Geometry check sheet. Reference: the model listing, model coordinates, mm. Give positions to 0.01 mm unless a question says otherwise; leave off trailing zeros. Write each loop counter-clockwise with the first axis right and the second up, starting at its lowest first coordinate (ties: lowest second). Pieces come first, ordered by that corner, then holes. Notation, with made-up numbers: (45, 46.5) -> (49, 46.5) arc R23 cw to (49, 84.5) -> close; hole circle Ø6 at (68, -35.5). An arc over 180 degrees is marked (long way). Write item = value, one per line. Start each with the question number.
1. Depth check by flat-ended pin: P1, Ø1.5, axis at x = -33, z = 1.5, coming from the +Y side; P2, Ø1.5, axis at x = -59, z = 1, coming from the -Y side. Enter the tip coordinate at first touch or a pass-through.
2. Cross-section at C-C, the plane z = 2.1. State how many separate pieces and enclosed holes the cut face has, plus the area to 3 significant figures.
3. Cross-section at B-B, the plane x = 27.5. Record the cut outline in (y, z).
4. Thickness scan on line 1 along X through (y, z) = (45.5, 0.8); line 2 along Y through (x, z) = (23.5, 2.65). Record the ranges inside material, lowest first.
5. Cross-section at A-A, the plane y = -53. Record the cut outline in (x, z), plus the area to 3 significant figures.
Autodesk Inventor part; units mm, degrees
ref_plane "YZ Plane" through (0, 0, 0) normal (1, 0, 0) x (0, 1, 0)
ref_plane "XZ Plane" through (0, 0, 0) normal (0, 1, 0) x (-1, 0, 0)
ref_plane "XY Plane" through (0, 0, 0) normal (0, 0, 1) x (1, 0, 0)
sketch "Sketch1" plane through (0, 0, 0) normal (0, 0, 1) x (1, 0, 0)
  line L0 (-65, -90.5) -> (65, -90.5)
  line L1 (65, -90.5) -> (65, 90.5)
  line L2 (65, 90.5) -> (-65, 90.5)
  line L3 (-65, 90.5) -> (-65, -90.5)
  line L4 (-65, -90.5) -> (65, 90.5) construction
  line L5 (65, -90.5) -> (-65, 90.5) construction
  line L6 (-60, 77.5) -> (-57, 77.5)
  line L7 (-57, 77.5) -> (-57, 62.5)
  line L8 (-57, 62.5) -> (-60, 62.5)
  line L9 (-60, 62.5) -> (-60, 77.5)
  line L10 (-60, 77.5) -> (-57, 62.5) construction
  line L11 (-57, 77.5) -> (-60, 62.5) construction
  line L12 (-60, 57.5) -> (-57, 57.5)
  line L13 (-57, 57.5) -> (-57, 42.5)
  line L14 (-57, 42.5) -> (-60, 42.5)
  line L15 (-60, 42.5) -> (-60, 57.5)
  line L16 (-60, 57.5) -> (-57, 42.5) construction
  line L17 (-57, 57.5) -> (-60, 42.5) construction
  line L18 (-60, 37.5) -> (-57, 37.5)
  line L19 (-57, 37.5) -> (-57, 22.5)
  line L20 (-57, 22.5) -> (-60, 22.5)
  line L21 (-60, 22.5) -> (-60, 37.5)
  line L22 (-60, 37.5) -> (-57, 22.5) construction
  line L23 (-57, 37.5) -> (-60, 22.5) construction
  line L24 (-60, 17.5) -> (-57, 17.5)
  line L25 (-57, 17.5) -> (-57, 2.5)
  line L26 (-57, 2.5) -> (-60, 2.5)
  line L27 (-60, 2.5) -> (-60, 17.5)
  line L28 (-60, 17.5) -> (-57, 2.5) construction
  line L29 (-57, 17.5) -> (-60, 2.5) construction
  line L30 (-60, -2.5) -> (-57, -2.5)
  line L31 (-57, -2.5) -> (-57, -17.5)
  line L32 (-57, -17.5) -> (-60, -17.5)
  line L33 (-60, -17.5) -> (-60, -2.5)
  line L34 (-60, -2.5) -> (-57, -17.5) construction
  line L35 (-57, -2.5) -> (-60, -17.5) construction
  line L36 (-60, -22.5) -> (-57, -22.5)
  line L37 (-57, -22.5) -> (-57, -37.5)
  line L38 (-57, -37.5) -> (-60, -37.5)
  line L39 (-60, -37.5) -> (-60, -22.5)
  line L40 (-60, -22.5) -> (-57, -37.5) construction
  line L41 (-57, -22.5) -> (-60, -37.5) construction
  line L42 (-60, -42.5) -> (-57, -42.5)
  line L43 (-57, -42.5) -> (-57, -57.5)
  line L44 (-57, -57.5) -> (-60, -57.5)
  line L45 (-60, -57.5) -> (-60, -42.5)
  line L46 (-60, -42.5) -> (-57, -57.5) construction
  line L47 (-57, -42.5) -> (-60, -57.5) construction
  line L48 (-60, -62.5) -> (-57, -62.5)
  line L49 (-57, -62.5) -> (-57, -77.5)
  line L50 (-57, -77.5) -> (-60, -77.5)
  line L51 (-60, -77.5) -> (-60, -62.5)
  line L52 (-60, -62.5) -> (-57, -77.5) construction
  line L53 (-57, -62.5) -> (-60, -77.5) construction
  line L54 (57, 77.5) -> (60, 77.5)
  line L55 (60, 77.5) -> (60, 62.5)
  line L56 (60, 62.5) -> (57, 62.5)
  line L57 (57, 62.5) -> (57, 77.5)
  line L58 (57, 77.5) -> (60, 62.5) construction
  line L59 (60, 77.5) -> (57, 62.5) construction
  line L60 (57, 57.5) -> (60, 57.5)
  line L61 (60, 57.5) -> (60, 42.5)
  line L62 (60, 42.5) -> (57, 42.5)
  line L63 (57, 42.5) -> (57, 57.5)
  line L64 (57, 57.5) -> (60, 42.5) construction
  line L65 (60, 57.5) -> (57, 42.5) construction
  line L66 (57, 37.5) -> (60, 37.5)
  line L67 (60, 37.5) -> (60, 22.5)
  line L68 (60, 22.5) -> (57, 22.5)
  line L69 (57, 22.5) -> (57, 37.5)
  line L70 (57, 37.5) -> (60, 22.5) construction
  line L71 (60, 37.5) -> (57, 22.5) construction
  line L72 (57, 17.5) -> (60, 17.5)
  line L73 (60, 17.5) -> (60, 2.5)
  line L74 (60, 2.5) -> (57, 2.5)
  line L75 (57, 2.5) -> (57, 17.5)
  line L76 (57, 17.5) -> (60, 2.5) construction
  line L77 (60, 17.5) -> (57, 2.5) construction
  line L78 (57, -2.5) -> (60, -2.5)
  line L79 (60, -2.5) -> (60, -17.5)
  line L80 (60, -17.5) -> (57, -17.5)
  line L81 (57, -17.5) -> (57, -2.5)
  line L82 (57, -2.5) -> (60, -17.5) construction
  line L83 (60, -2.5) -> (57, -17.5) construction
  line L84 (57, -22.5) -> (60, -22.5)
  line L85 (60, -22.5) -> (60, -37.5)
  line L86 (60, -37.5) -> (57, -37.5)
  line L87 (57, -37.5) -> (57, -22.5)
  line L88 (57, -22.5) -> (60, -37.5) construction
  line L89 (60, -22.5) -> (57, -37.5) construction
  line L90 (57, -42.5) -> (60, -42.5)
  line L91 (60, -42.5) -> (60, -57.5)
  line L92 (60, -57.5) -> (57, -57.5)
  line L93 (57, -57.5) -> (57, -42.5)
  line L94 (57, -42.5) -> (60, -57.5) construction
  line L95 (60, -42.5) -> (57, -57.5) construction
  line L96 (57, -62.5) -> (60, -62.5)
  line L97 (60, -62.5) -> (60, -77.5)
  line L98 (60, -77.5) -> (57, -77.5)
  line L99 (57, -77.5) -> (57, -62.5)
  line L100 (57, -62.5) -> (60, -77.5) construction
  line L101 (60, -62.5) -> (57, -77.5) construction
  point P0 (0, 0)
  point P1 (-58.5, 70)
  point P2 (-58.5, 50)
  point P3 (-58.5, 30)
  point P4 (-58.5, 10)
  point P5 (-58.5, -10)
  point P6 (-58.5, -30)
  point P7 (-58.5, -50)
  point P8 (-58.5, -70)
  point P9 (58.5, 70)
  point P10 (58.5, 50)
  point P11 (58.5, 30)
  point P12 (58.5, 10)
  point P13 (58.5, -10)
  point P14 (58.5, -30)
  point P15 (58.5, -50)
  point P16 (58.5, -70)
  dimension "d0" = 130
  dimension "d1" = 181
  dimension "d2" = 3
  dimension "d3" = 15
  dimension "d8" = 5
  dimension "d9" = 13
  dimension "d12" = 20
  dimension "d15" = 117
extrude "Extrusion1" add sketch "Sketch1" along normal blind 3
sketch "Sketch2" plane through (0, 0, 3) normal (0, 0, 1) x (1, 0, 0)
  line L0 (65, 90.5) -> (-65, 90.5)
  line L1 (-52.5, 90.5) -> (-37.5, 90.5)
  line L2 (-37.5, 90.5) -> (-37.5, 93.5)
  line L3 (-37.5, 93.5) -> (-52.5, 93.5)
  line L4 (-52.5, 93.5) -> (-52.5, 90.5)
  line L5 (-22.5, 90.5) -> (-7.5, 90.5)
  line L6 (-7.5, 90.5) -> (-7.5, 93.5)
  line L7 (-7.5, 93.5) -> (-22.5, 93.5)
  line L8 (-22.5, 93.5) -> (-22.5, 90.5)
  line L9 (7.5, 90.5) -> (22.5, 90.5)
  line L10 (22.5, 90.5) -> (22.5, 93.5)
  line L11 (22.5, 93.5) -> (7.5, 93.5)
  line L12 (7.5, 93.5) -> (7.5, 90.5)
  line L13 (37.5, 90.5) -> (52.5, 90.5)
  line L14 (52.5, 90.5) -> (52.5, 93.5)
  line L15 (52.5, 93.5) -> (37.5, 93.5)
  line L16 (37.5, 93.5) -> (37.5, 90.5)
  line L17 (-52.5, -93.5) -> (-37.5, -93.5)
  line L18 (-37.5, -93.5) -> (-37.5, -90.5)
  line L19 (-37.5, -90.5) -> (-52.5, -90.5)
  line L20 (-52.5, -90.5) -> (-52.5, -93.5)
  line L21 (-22.5, -93.5) -> (-7.5, -93.5)
  line L22 (-7.5, -93.5) -> (-7.5, -90.5)
  line L23 (-7.5, -90.5) -> (-22.5, -90.5)
  line L24 (-22.5, -90.5) -> (-22.5, -93.5)
  line L25 (7.5, -93.5) -> (22.5, -93.5)
  line L26 (22.5, -93.5) -> (22.5, -90.5)
  line L27 (22.5, -90.5) -> (7.5, -90.5)
  line L28 (7.5, -90.5) -> (7.5, -93.5)
  line L29 (37.5, -93.5) -> (52.5, -93.5)
  line L30 (52.5, -93.5) -> (52.5, -90.5)
  line L31 (52.5, -90.5) -> (37.5, -90.5)
  line L32 (37.5, -90.5) -> (37.5, -93.5)
  line L33 (-65, 90.5) -> (-65, -90.5)
  point P0 (0, 0)
  dimension "d20" = 15
  dimension "d21" = 3
  dimension "d24" = 30
  dimension "d27" = 184
  dimension "d30" = 12.5
extrude "Extrusion2" add sketch "Sketch2" against normal blind 3
equation "\"BendRadius\" = Thickness"
equation "\"BendReliefWidth\" = Thickness"
equation "\"BendReliefDepth\" = 0.5 * Thickness"
equation "\"CornerReliefSize\" = 4 * Thickness"
equation "\"MinimumRemnant\" = 2 * Thickness"
equation "\"TransitionRadius\" = BendRadius"
equation "\"JacobiRadiusSize\" = BendRadius"
equation "\"GapSize\" = Thickness"
properties part number "1 binnen achterplaat"
Answers:
q1.P1 = 90.5
q1.P2 = -90.5
q2.separate_pieces = 1
q2.enclosed_holes = 16
q2.area = 23,200 mm^2
q3.outline = (-90.5, 0) -> (90.5, 0) -> (90.5, 3) -> (-90.5, 3) -> close
q4.line_1 = -65 to -60, -57 to 57, 60 to 65
q4.line_2 = -90.5 to 90.5
q5.outline = (-65, 0) -> (-60, 0) -> (-60, 3) -> (-65, 3) -> close; (-57, 0) -> (57, 0) -> (57, 3) -> (-57, 3) -> close; (60, 0) -> (65, 0) -> (65, 3) -> (60, 3) -> close
q5.area = 372 mm^2
